Build history of the part. All positions in model axes, mm. A direction names the side the tool comes from. Coordinates: 2 decimals unless noted, no trailing zeros. Write each loop counter-clockwise with the first axis right and the second up, starting at its lowest first coordinate (ties: lowest second). Pieces come first, ordered by that corner, then holes. Notation, with made-up numbers: M -19,17 L 1,17 A21 cw 1,52 Z; hole C -35,37 d8. An arc over 180 degrees is marked long. Use CSV: the item, a comma, the result in double quotes. Start each with the question number.
```python
from build123d import *

# Parameters (mm, degrees)
CUT_EXTRUDE1_REACH = 10
CUT_EXTRUDE2_REACH = 10


with BuildPart() as part:
    # Sketch1 → Revolve3 (revolve)
    with BuildSketch(Plane.XY):
        Polygon((40, 4), (37, 4), (17.5, 4), (17.5, 3), (10, 3), (10, 4), (0, 4), (0, -4), (10, -4), (10, -3), (17.5, -3), (17.5, -4), (37, -4), (40, -4), (40, -3.5), (38, -3.5), (38, 3.5), (40, 3.5), align=None)
    revolve(axis=Axis((0, 4, 0), (0, -1, 0)))

    # Sketch2 → Cut-Extrude1 (cut, up to next)
    with BuildSketch(Plane(origin=(0, 4, 0), x_dir=(1, 0, 0), z_dir=(0, 1, 0)), mode=Mode.PRIVATE) as cut_extrude1_sk1:
        with BuildLine():
            ThreePointArc((2.5, 0), (1.118033989, 2.236067977), (-1.5, 2))
            Line((-1.5, 2), (-1.5, -2))
            ThreePointArc((-1.5, -2), (1.118033989, -2.236067977), (2.5, 0))
        make_face()
    cut_extrude1_tool1 = extrude(cut_extrude1_sk1.sketch, amount=-CUT_EXTRUDE1_REACH, mode=Mode.PRIVATE) & part.part
    add(cut_extrude1_tool1.solids().sort_by_distance((0.316718, 4, 0))[0], mode=Mode.SUBTRACT)

    # Sketch3 → Cut-Extrude2 (cut, up to next)
    with BuildSketch(Plane(origin=(0, 4, 0), x_dir=(1, 0, 0), z_dir=(0, 1, 0)), mode=Mode.PRIVATE) as cut_extrude2_sk1:
        with BuildLine():
            Line((4.553448892, -20.475988454), (6.725889759, -30.245039378))
            ThreePointArc((6.725889759, -30.245039378), (6.584709324, -31.012405912), (5.935210643, -31.444765457))
            ThreePointArc((5.935210643, -31.444765457), (-1.374941712, -31.970447843), (-8.612970493, -30.81909699))
            ThreePointArc((-8.612970493, -30.81909699), (-9.22295101, -30.33257147), (-9.297728295, -29.555917319))
            Line((-9.297728295, -29.555917319), (-6.294591812, -20.009450615))
            ThreePointArc((-6.294591812, -20.009450615), (-5.823993451, -19.434086857), (-5.08636065, -19.342412862))
            ThreePointArc((-5.08636065, -19.342412862), (-0.85933857, -19.981529902), (3.406947089, -19.707681536))
            ThreePointArc((3.406947089, -19.707681536), (4.133985694, -19.862346135), (4.553448892, -20.475988454))
        make_face()
    cut_extrude2_tool1 = extrude(cut_extrude2_sk1.sketch, amount=-CUT_EXTRUDE2_REACH, mode=Mode.PRIVATE) & part.part
    add(cut_extrude2_tool1.solids().sort_by_distance((-1.124173, 4, 26.139518))[0], mode=Mode.SUBTRACT)
    # Sketch3 → Cut-Extrude2 (cut, up to next)
    with BuildSketch(Plane(origin=(0, 4, 0), x_dir=(1, 0, 0), z_dir=(0, 1, 0)), mode=Mode.PRIVATE) as cut_extrude2_sk2:
        with BuildLine():
            Line((-18.599766773, -9.697869663), (-27.473676287, -14.324702834))
            ThreePointArc((-27.473676287, -14.324702834), (-27.969978179, -14.926755776), (-27.882682314, -15.70210263))
            ThreePointArc((-27.882682314, -15.70210263), (-23.578751076, -21.634289859), (-18.037979194, -26.431634581))
            ThreePointArc((-18.037979194, -26.431634581), (-17.272989906, -26.585175136), (-16.630550183, -26.142394699))
            Line((-16.630550183, -26.142394699), (-11.258935698, -17.698484877))
            ThreePointArc((-11.258935698, -17.698484877), (-11.121630324, -16.96796896), (-11.526359866, -16.344510646))
            ThreePointArc((-11.526359866, -16.344510646), (-14.736719422, -13.521431162), (-17.273751407, -10.080551193))
            ThreePointArc((-17.273751407, -10.080551193), (-17.860159866, -9.62378934), (-18.599766773, -9.697869663))
        make_face()
    cut_extrude2_tool2 = extrude(cut_extrude2_sk2.sketch, amount=-CUT_EXTRUDE2_REACH, mode=Mode.PRIVATE) & part.part
    add(cut_extrude2_tool2.solids().sort_by_distance((-19.278341, 4, 17.68852))[0], mode=Mode.SUBTRACT)
    # Sketch3 → Cut-Extrude2 (cut, up to next)
    with BuildSketch(Plane(origin=(0, 4, 0), x_dir=(1, 0, 0), z_dir=(0, 1, 0)), mode=Mode.PRIVATE) as cut_extrude2_sk3:
        with BuildLine():
            Line((-20.009450615, 6.294591812), (-29.555917319, 9.297728295))
            ThreePointArc((-29.555917319, 9.297728295), (-30.33257147, 9.22295101), (-30.81909699, 8.612970493))
            ThreePointArc((-30.81909699, 8.612970493), (-31.970447843, 1.374941712), (-31.444765457, -5.935210643))
            ThreePointArc((-31.444765457, -5.935210643), (-31.012405912, -6.584709324), (-30.245039378, -6.725889759))
            Line((-30.245039378, -6.725889759), (-20.475988454, -4.553448892))
            ThreePointArc((-20.475988454, -4.553448892), (-19.862346135, -4.133985694), (-19.707681536, -3.406947089))
            ThreePointArc((-19.707681536, -3.406947089), (-19.981529902, 0.85933857), (-19.342412862, 5.08636065))
            ThreePointArc((-19.342412862, 5.08636065), (-19.434086857, 5.823993451), (-20.009450615, 6.294591812))
        make_face()
    cut_extrude2_tool3 = extrude(cut_extrude2_sk3.sketch, amount=-CUT_EXTRUDE2_REACH, mode=Mode.PRIVATE) & part.part
    add(cut_extrude2_tool3.solids().sort_by_distance((-26.139518, 4, -1.124173))[0], mode=Mode.SUBTRACT)
    # Sketch3 → Cut-Extrude2 (cut, up to next)
    with BuildSketch(Plane(origin=(0, 4, 0), x_dir=(1, 0, 0), z_dir=(0, 1, 0)), mode=Mode.PRIVATE) as cut_extrude2_sk4:
        with BuildLine():
            Line((-9.697869663, 18.599766773), (-14.324702834, 27.473676287))
            ThreePointArc((-14.324702834, 27.473676287), (-14.926755776, 27.969978179), (-15.70210263, 27.882682314))
            ThreePointArc((-15.70210263, 27.882682314), (-21.634289859, 23.578751076), (-26.431634581, 18.037979194))
            ThreePointArc((-26.431634581, 18.037979194), (-26.585175136, 17.272989906), (-26.142394699, 16.630550183))
            Line((-26.142394699, 16.630550183), (-17.698484877, 11.258935698))
            ThreePointArc((-17.698484877, 11.258935698), (-16.96796896, 11.121630324), (-16.344510646, 11.526359866))
            ThreePointArc((-16.344510646, 11.526359866), (-13.521431162, 14.736719422), (-10.080551193, 17.273751407))
            ThreePointArc((-10.080551193, 17.273751407), (-9.62378934, 17.860159866), (-9.697869663, 18.599766773))
        make_face()
    cut_extrude2_tool4 = extrude(cut_extrude2_sk4.sketch, amount=-CUT_EXTRUDE2_REACH, mode=Mode.PRIVATE) & part.part
    add(cut_extrude2_tool4.solids().sort_by_distance((-17.68852, 4, -19.278341))[0], mode=Mode.SUBTRACT)
    # Sketch3 → Cut-Extrude2 (cut, up to next)
    with BuildSketch(Plane(origin=(0, 4, 0), x_dir=(1, 0, 0), z_dir=(0, 1, 0)), mode=Mode.PRIVATE) as cut_extrude2_sk5:
        with BuildLine():
            Line((6.294591812, 20.009450615), (9.297728295, 29.555917319))
            ThreePointArc((9.297728295, 29.555917319), (9.22295101, 30.33257147), (8.612970493, 30.81909699))
            ThreePointArc((8.612970493, 30.81909699), (1.374941712, 31.970447843), (-5.935210643, 31.444765457))
            ThreePointArc((-5.935210643, 31.444765457), (-6.584709324, 31.012405912), (-6.725889759, 30.245039378))
            Line((-6.725889759, 30.245039378), (-4.553448892, 20.475988454))
            ThreePointArc((-4.553448892, 20.475988454), (-4.133985694, 19.862346135), (-3.406947089, 19.707681536))
            ThreePointArc((-3.406947089, 19.707681536), (0.85933857, 19.981529902), (5.08636065, 19.342412862))
            ThreePointArc((5.08636065, 19.342412862), (5.823993451, 19.434086857), (6.294591812, 20.009450615))
        make_face()
    cut_extrude2_tool5 = extrude(cut_extrude2_sk5.sketch, amount=-CUT_EXTRUDE2_REACH, mode=Mode.PRIVATE) & part.part
    add(cut_extrude2_tool5.solids().sort_by_distance((1.124173, 4, -26.139518))[0], mode=Mode.SUBTRACT)
    # Sketch3 → Cut-Extrude2 (cut, up to next)
    with BuildSketch(Plane(origin=(0, 4, 0), x_dir=(1, 0, 0), z_dir=(0, 1, 0)), mode=Mode.PRIVATE) as cut_extrude2_sk6:
        with BuildLine():
            Line((18.599766773, 9.697869663), (27.473676287, 14.324702834))
            ThreePointArc((27.473676287, 14.324702834), (27.969978179, 14.926755776), (27.882682314, 15.70210263))
            ThreePointArc((27.882682314, 15.70210263), (23.578751076, 21.634289859), (18.037979194, 26.431634581))
            ThreePointArc((18.037979194, 26.431634581), (17.272989906, 26.585175136), (16.630550183, 26.142394699))
            Line((16.630550183, 26.142394699), (11.258935698, 17.698484877))
            ThreePointArc((11.258935698, 17.698484877), (11.121630324, 16.96796896), (11.526359866, 16.344510646))
            ThreePointArc((11.526359866, 16.344510646), (14.736719422, 13.521431162), (17.273751407, 10.080551193))
            ThreePointArc((17.273751407, 10.080551193), (17.860159866, 9.62378934), (18.599766773, 9.697869663))
        make_face()
    cut_extrude2_tool6 = extrude(cut_extrude2_sk6.sketch, amount=-CUT_EXTRUDE2_REACH, mode=Mode.PRIVATE) & part.part
    add(cut_extrude2_tool6.solids().sort_by_distance((19.278341, 4, -17.68852))[0], mode=Mode.SUBTRACT)
    # Sketch3 → Cut-Extrude2 (cut, up to next)
    with BuildSketch(Plane(origin=(0, 4, 0), x_dir=(1, 0, 0), z_dir=(0, 1, 0)), mode=Mode.PRIVATE) as cut_extrude2_sk7:
        with BuildLine():
            Line((20.009450615, -6.294591812), (29.555917319, -9.297728295))
            ThreePointArc((29.555917319, -9.297728295), (30.33257147, -9.22295101), (30.81909699, -8.612970493))
            ThreePointArc((30.81909699, -8.612970493), (31.970447843, -1.374941712), (31.444765457, 5.935210643))
            ThreePointArc((31.444765457, 5.935210643), (31.012405912, 6.584709324), (30.245039378, 6.725889759))
            Line((30.245039378, 6.725889759), (20.475988454, 4.553448892))
            ThreePointArc((20.475988454, 4.553448892), (19.862346135, 4.133985694), (19.707681536, 3.406947089))
            ThreePointArc((19.707681536, 3.406947089), (19.981529902, -0.85933857), (19.342412862, -5.08636065))
            ThreePointArc((19.342412862, -5.08636065), (19.434086857, -5.823993451), (20.009450615, -6.294591812))
        make_face()
    cut_extrude2_tool7 = extrude(cut_extrude2_sk7.sketch, amount=-CUT_EXTRUDE2_REACH, mode=Mode.PRIVATE) & part.part
    add(cut_extrude2_tool7.solids().sort_by_distance((26.139518, 4, 1.124173))[0], mode=Mode.SUBTRACT)
    # Sketch3 → Cut-Extrude2 (cut, up to next)
    with BuildSketch(Plane(origin=(0, 4, 0), x_dir=(1, 0, 0), z_dir=(0, 1, 0)), mode=Mode.PRIVATE) as cut_extrude2_sk8:
        with BuildLine():
            Line((9.697869663, -18.599766773), (14.324702834, -27.473676287))
            ThreePointArc((14.324702834, -27.473676287), (14.926755776, -27.969978179), (15.70210263, -27.882682314))
            ThreePointArc((15.70210263, -27.882682314), (21.634289859, -23.578751076), (26.431634581, -18.037979194))
            ThreePointArc((26.431634581, -18.037979194), (26.585175136, -17.272989906), (26.142394699, -16.630550183))
            Line((26.142394699, -16.630550183), (17.698484877, -11.258935698))
            ThreePointArc((17.698484877, -11.258935698), (16.96796896, -11.121630324), (16.344510646, -11.526359866))
            ThreePointArc((16.344510646, -11.526359866), (13.521431162, -14.736719422), (10.080551193, -17.273751407))
            ThreePointArc((10.080551193, -17.273751407), (9.62378934, -17.860159866), (9.697869663, -18.599766773))
        make_face()
    cut_extrude2_tool8 = extrude(cut_extrude2_sk8.sketch, amount=-CUT_EXTRUDE2_REACH, mode=Mode.PRIVATE) & part.part
    add(cut_extrude2_tool8.solids().sort_by_distance((17.68852, 4, 19.278341))[0], mode=Mode.SUBTRACT)


solid = part.part
```
1. Flat gauge pins, fed straight in: pin 1 (4.5 mm diameter, centred on y = 1.5, z = -0.5, fed in from +X); pin 2 (2 mm diameter, centred on x = -10, z = -8.5, fed in from -Y); pin 3 (1.5 mm diameter, centred on y = 0, z = -7.5, fed in from +X). Where does each tip first touch, or does it go through?
2. Slice it at A-A (x = 21.5). List the corners of the cut face in (y, z), and give its area (3 significant figures).
3. Slice it at B-B (y = -0.5). Count the separate pieces of the cut face and the enclosed holes in it, and give its area (3 significant figures).
4. Slice it at C-C (x = -34.5). List the corners of the cut face in (y, z), and give its area (3 significant figures).
5. 3-axis set-ups, long thin cutter, end or side, ignore diameter. For faces 4 (the flat face through (-8, -3, -8)), 5 (the cylindrical face through (-13.887, 3.493, -10.648)), 6 (the cylindrical face through (23.648, 0.056, -21.558)): which of +Z, -Z, +X, -X, +Y, -Y reach the whole face in a straight line?
6. Pull direction X, two halves, no side cores. Call faces 1 (the flat face through (24.716, 0.056, 7.775)), 2 (the cylindrical face through (17.535, 0.049, -33.713)), 3 (the flat face through (35.4, -3.5, -14.6)): pulls with the +X half, pulls with the -X half, needs draft (parallel to the pull), parting line crosses it, or undercut.
7. Drill centre lines: line 1 along Z through (x, y) = (0, 3.3); line 2 along Z through (x, y) = (0, 3.8); line 3 along Z through (x, y) = (-13.5, 1.5). Where is each one in solid material? Low to high. Write a range as from..to.
Established:
1,pin 1,"stops at x = 40"
1,pin 2,"stops at y = -3"
1,pin 3,"stops at x = 37.4"
2,outline,"M -4,-33.73 L -3.5,-33.73 L -3.5,-31.33 L 3.5,-31.33 L 3.5,-33.73 L 4,-33.73 L 4,-23.7 L -4,-23.7 Z; M -4,-11.21 L 4,-11.21 L 4,-4.78 L -4,-4.78 Z; M -4,6.76 L 4,6.76 L 4,13.68 L -4,13.68 Z; M -4,23.7 L 4,23.7 L 4,33.73 L 3.5,33.73 L 3.5,31.33 L -3.5,31.33 L -3.5,33.73 L -4,33.73 Z"
2,area,"234 mm2"
3,separate pieces,"1"
3,enclosed holes,"9"
3,area,"3,220 mm2"
4,outline,"M -4,-20.24 L -3.5,-20.24 L -3.5,-15.93 L 3.5,-15.93 L 3.5,-20.24 L 4,-20.24 L 4,20.24 L 3.5,20.24 L 3.5,15.93 L -3.5,15.93 L -3.5,20.24 L -4,20.24 Z"
4,area,"263 mm2"
5,face 4,"-Y"
5,face 5,"+Y"
5,face 6,"+Y, -Y"
6,face 1,"undercut"
6,face 2,"parting line crosses it"
6,face 3,"needs draft"
7,line 1,"z = -38..-32, -20..-17.5, -10..-2.5, 2.5..10, 17.5..20, 32..38"
7,line 2,"z = -40..-32, -20..-17.5, -10..-2.5, 2.5..10, 17.5..20, 32..40"
7,line 3,"z = -35.52..-25.89, -14.76..14.76, 21.22..35.52"
